Work out the finished part from the listing and answer in its coordinate system (mm). A direction names the side the tool comes from. Coordinates: 2 decimals unless noted, no trailing zeros. Order: outer loops, then holes, each group sorted by start corner. A loop starts at its lowest first (then second) coordinate and runs counter-clockwise, first axis right, second up. Notation, with made-up numbers: (73.25, 67.25) - (120.25, 67.25) arc R23 cw to (120.25, 99.25) - close; hole circle Ø7 at (55, -5.5). An arc over 180 degrees is marked (long way). Answer as a JSON object with one key per item and string values. Group by question number.
1) Section A-A (x = 0) is taken. Give the vertices of the cut face in (y, z).
2) Section C-C (z = 0) is taken. Give the vertices of the cut face in (x, y), plus the area to 3 significant figures.
3) Each of these flat-tipped pins is pushed along its axis until it touches: P1, Ø9, axis at x = 0, z = 0, coming from the +Y side; P2, Ø3, axis at y = 10.5, z = -1.5, coming from the -X side; P3, Ø4, axis at x = -6, y = 11, coming from the +Z side. Where does it stop, or does it pass through?
4) Find the intervals of material crossed by line 1 along X through (y, z) = (10.5, 0); line 2 along X through (y, z) = (27.25, 0); line 3 along Y through (x, z) = (-4.25, 1), in increasing order.
5) The mould has two halves that part along X. Classify faces 4 (the face through (0.33, 22.888, -7.493)), 5 (the face through (0, 15, 0)), 6 (the face through (-3.92, 0, -1.42)): released by +X, released by -X, zero draft, split by the parting line, or undercut.
6) A tool of negligible diameter and unlimited length cuts with its end or side. For faces 1 (the face through (2, 31, 5)), 2 (the face through (-3.905, 7.395, -0.867)), 3 (the face through (-5.028, 26.07, -1.116)), from which of +Z, -Z, +X, -X, +Y, -Y can it reach the whole face along a straight path? Write none if from no direction.
7) Section D-D (y = 23.5) is taken. Give the vertices of the cut face in (x, z).
8) Section B-B (y = 4) is taken. Give the vertices of the cut face in (x, z), plus the area to 3 significant figures.
from build123d import *

# Parameters (mm, degrees)
SKETCH1_R           = 6
SKETCH1_R_2         = 4
BOSS_EXTRUDE1_DEPTH = 15
SKETCH2_R           = 7.5
BOSS_EXTRUDE2_DEPTH = 16
FILLET1_R           = 5
SKETCH3_R           = 5.15
CUT_EXTRUDE1_DEPTH  = 10


with BuildPart() as part:
    # Sketch1 → Boss-Extrude1 (new body)
    with BuildSketch(Plane(origin=(0, 0, 0), x_dir=(1, 0, 0), z_dir=(0, 1, 0))):
        with Locations(Location((0, 0, 0), (0, 0, 270))):
            Circle(SKETCH1_R)
        with Locations(Location((0, 0, 0), (0, 0, 270))):
            Circle(SKETCH1_R_2, mode=Mode.SUBTRACT)
    extrude(amount=BOSS_EXTRUDE1_DEPTH)

    # Sketch2 → Boss-Extrude2 (add)
    with BuildSketch(Plane(origin=(0, 15, 0), x_dir=(1, 0, 0), z_dir=(0, 1, 0))):
        with Locations(Location((0, 0, 0), (0, 0, 270))):
            Circle(SKETCH2_R)
    extrude(amount=BOSS_EXTRUDE2_DEPTH)

    # Fillet1
    # the kernel refuses this fillet: 5 mm, written as the material it adds along each edge
    with BuildSketch(Plane(origin=(0, 15, 0), x_dir=(0, 0, 1), z_dir=(-1, 0, 0))) as fillet1_piece_1:
        with BuildLine():
            CenterArc((11, -3.570714214), FILLET1_R, 134.427004001, 45.572995999)
            Line((6, -3.570714214), (5.9, -3.570714214))
            Line((5.9, -3.570714214), (5.9, 0))
            Line((5.9, 0), (6, 0.1))
            ThreePointArc((6, 0.1), (6.75, 0.1), (7.43, 0.071414284))
            Line((7.43, 0.071414284), (7.5, 0))
        make_face()
    revolve(axis=Axis((0, 15, 0), (0, 1, 0)))

    # Sketch3 → Cut-Extrude1 (cut)
    with BuildSketch(Plane(origin=(0, 31, 0), x_dir=(1, 0, 0), z_dir=(0, 1, 0))):
        with Locations(Location((0, 0, 0), (0, 0, 270))):
            Circle(SKETCH3_R)
    extrude(amount=-CUT_EXTRUDE1_DEPTH, mode=Mode.SUBTRACT)


solid = part.part
Report:
{
 "1": {"outline": "(0, -6) - (11.43, -6) arc R5 cw to (15, -7.5) - (31, -7.5) - (31, -5.15) - (21, -5.15) - (21, 5.15) - (31, 5.15) - (31, 7.5) - (15, 7.5) arc R5 cw to (11.43, 6) - (0, 6) - (0, 4) - (15, 4) - (15, -4) - (0, -4) - close"},
 "2": {"outline": "(-7.5, 15) arc R5 cw to (-6, 11.43) - (-6, 0) - (-4, 0) - (-4, 15) - (4, 15) - (4, 0) - (6, 0) - (6, 11.43) arc R5 cw to (7.5, 15) - (7.5, 31) - (5.15, 31) - (5.15, 21) - (-5.15, 21) - (-5.15, 31) - (-7.5, 31) - close", "area": "200 mm²"},
 "3": {"P1": "stops at y = 21", "P2": "stops at x = -6", "P3": "stops at z = 4.47"},
 "4": {"line 1": "x = -6 to -4, 4 to 6", "line 2": "x = -7.5 to -5.15, 5.15 to 7.5", "line 3": "y = 0 to 21"},
 "5": {"face 4": "split by the parting line", "face 5": "undercut", "face 6": "zero draft"},
 "6": {"face 1": "+Z, -Z, +X, -X, +Y", "face 2": "-Y", "face 3": "+Y"},
 "7": {"outline": "circle Ø15 at (0, 0); hole circle Ø10.3 at (0, 0)"},
 "8": {"outline": "circle Ø12 at (0, 0); hole circle Ø8 at (0, 0)", "area": "62.8 mm²"}
}
